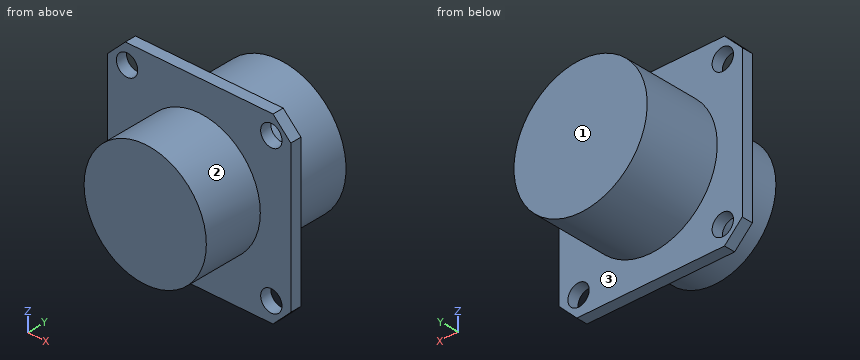
```python
from build123d import *

# Parameters (mm, degrees)
SKETCH1_W           = 26.1874
SKETCH1_H           = 26.1874
BOSS_EXTRUDE1_DEPTH = 1.5875
CHAMFER1_SIZE       = 2.54
SKETCH2_R           = 1.524
CUT_EXTRUDE1_DEPTH  = 19.585212284
SKETCH3_R           = 9.525
BOSS_EXTRUDE2_DEPTH = 10.9474
SKETCH4_R           = 8.7376
BOSS_EXTRUDE3_DEPTH = 8.4328


with BuildPart() as part:
    # Sketch1 → Boss-Extrude1 (new body)
    with BuildSketch(Plane(origin=(0, 0, 0), x_dir=(1, 0, 0), z_dir=(0, 1, 0))):
        Rectangle(SKETCH1_W, SKETCH1_H)
    extrude(amount=BOSS_EXTRUDE1_DEPTH)

    # Chamfer1
    chamfer1_edges = [part.edges().sort_by_distance(p)[0] for p in [
        (13.0937, 0.79375, 13.0937),
        (-13.0937, 0.79375, 13.0937),
        (-13.0937, 0.79375, -13.0937),
        (13.0937, 0.79375, -13.0937),
    ]]
    chamfer(chamfer1_edges, length=CHAMFER1_SIZE)

    # Sketch2 → Cut-Extrude1 (cut, through all)
    with BuildSketch(Plane(origin=(0, 1.5875, 0), x_dir=(1, 0, 0), z_dir=(0, 1, 0))):
        with Locations(Location((-10.3124, 10.3124, 0), (0, 0, 270))):
            Circle(SKETCH2_R)
        with Locations(Location((10.3124, 10.3124, 0), (0, 0, 270))):
            Circle(SKETCH2_R)
        with Locations(Location((10.3124, -10.3124, 0), (0, 0, 270))):
            Circle(SKETCH2_R)
        with Locations(Location((-10.3124, -10.3124, 0), (0, 0, 270))):
            Circle(SKETCH2_R)
    extrude(amount=-CUT_EXTRUDE1_DEPTH, mode=Mode.SUBTRACT)

    # Sketch3 → Boss-Extrude2 (add)
    with BuildSketch(Plane(origin=(0, 1.5875, 0), x_dir=(1, 0, 0), z_dir=(0, 1, 0))):
        with Locations(Location((0, 0, 0), (0, 0, 270))):
            Circle(SKETCH3_R)
    extrude(amount=BOSS_EXTRUDE2_DEPTH)

    # Sketch4 → Boss-Extrude3 (add)
    with BuildSketch(Plane.XZ):
        with Locations(Location((0, 0, 0), (0, 0, 90))):
            Circle(SKETCH4_R)
    extrude(amount=BOSS_EXTRUDE3_DEPTH)


solid = part.part
```
Source: CAD feature listing. Evaluate the final solid. Frame: model axes, mm. Face numbers are marked on the shaded views. A direction names the side the tool comes from. Round coordinates to 2 decimals unless told otherwise and drop trailing zeros. Loops run counter-clockwise (first coordinate to the right, second up) from the corner with the lowest first, then second, coordinate; pieces in that order, holes last.
1. Section query A-A on x = 0. Output: boundary loops of the cut face in (y, z) (1 decimal).
2. Ray query, L1, parallel to Z at x = 11.25, y = 1; L2, parallel to Z at x = 11.5, y = 1; L3, parallel to Y at x = -4.5, z = 7.75. Return the intervals inside material, ascending.
3. Access query for the marked faces 1, 2 and 3. Directions: +Z, -Z, +X, -X, +Y, -Y. A direction counts if a zero-diameter tool reaches every point of the face in a straight line with its end or side. Return the directions, or none.
4. Section query B-B on z = 11. Output: boundary loops of the cut face in (x, y).
5. Section query C-C on y = 0.75. Output: boundary loops of the cut face in (x, z), and give its area (3 significant figures).
6. Contact query for flat-ended pins moving along their axis: pin 1 (4 mm diameter, centred on x = -8.5, z = 10, fed in from +Y); pin 2 (1.8 mm diameter, centred on x = -10.31, z = 10.31, fed in from -Y); pin 3 (2 mm diameter, centred on x = 3, y = -1.5, fed in from +Z); pin 4 (6 mm diameter, centred on x = 0.5, y = -3.5, fed in from -Z). Output: stop coordinate, or through.
7. Section query D-D on z = 0. Output: boundary loops of the cut face in (x, y) (1 decimal).
Answers below:
1. outline: (-8.4, -8.7) - (0, -8.7) - (0, -13.1) - (1.6, -13.1) - (1.6, -9.5) - (12.5, -9.5) - (12.5, 9.5) - (1.6, 9.5) - (1.6, 13.1) - (0, 13.1) - (0, 8.7) - (-8.4, 8.7) - close
2. L1: z = -12.4 to -11.51, -9.11 to 9.11, 11.51 to 12.4
2. L2: z = -12.15 to -11.27, -9.36 to 9.36, 11.27 to 12.15
2. L3: y = 0 to 12.53
3. face 1: +Z, -Z, +X, -X, +Y
3. face 2: -Y
3. face 3: +Y
4. outline: (-12.65, 0) - (-11.67, 0) - (-11.67, 1.59) - (-12.65, 1.59) - close; (-8.95, 0) - (8.95, 0) - (8.95, 1.59) - (-8.95, 1.59) - close; (11.67, 0) - (12.65, 0) - (12.65, 1.59) - (11.67, 1.59) - close
5. outline: (-13.09, -10.55) - (-10.55, -13.09) - (10.55, -13.09) - (13.09, -10.55) - (13.09, 10.55) - (10.55, 13.09) - (-10.55, 13.09) - (-13.09, 10.55) - close; hole circle Ø3.05 at (-10.31, -10.31); hole circle Ø3.05 at (-10.31, 10.31); hole circle Ø3.05 at (10.31, -10.31); hole circle Ø3.05 at (10.31, 10.31)
5. area: 644 mm2
6. pin 1: stops at y = 1.59
6. pin 2: passes through
6. pin 3: stops at z = 8.51
6. pin 4: stops at z = -8.74
7. outline: (-13.1, 0) - (-8.7, 0) - (-8.7, -8.4) - (8.7, -8.4) - (8.7, 0) - (13.1, 0) - (13.1, 1.6) - (9.5, 1.6) - (9.5, 12.5) - (-9.5, 12.5) - (-9.5, 1.6) - (-13.1, 1.6) - close
